Build history of the part. All positions in model axes, mm. A direction names the side the tool comes from. Coordinates: 2 decimals unless noted, no trailing zeros. Order: outer loops, then holes, each group sorted by start corner. A loop starts at its lowest first (then second) coordinate and runs counter-clockwise, first axis right, second up. Notation, with made-up numbers: (85.25, 30.25) -> (102.25, 30.25) arc R29 cw to (102.25, 63.25) -> close; hole circle Ø3 at (25.25, -8). An arc over 180 degrees is marked (long way). Write each question's results on one line, items separated by ' | '.
from build123d import *

# Parameters (mm, degrees)
F1_DEPTH      = 25.4
F1_DEPTH_BACK = 25.4
F2_W          = 21.4085327461
F2_H          = 21.4085327461
F3_DEPTH      = 25.4


with BuildPart() as f1:
    # F0 (on Front) → F1 (new body, two sides)
    with BuildSketch(Plane.XZ) as f1_sk:
        Polygon((0, 48.854034394), (0, 0), (77.7433076873, 0), (77.7433076873, 48.854034394), (56.3347749412, 48.854034394), (56.3347749412, 13.927792199), (21.4085327461, 13.927792199), (21.4085327461, 48.854034394), align=None)
    extrude(amount=F1_DEPTH)
    extrude(f1_sk.sketch, amount=-F1_DEPTH_BACK)

    # F2 (on face) → F3 (cut)
    with BuildSketch(Plane.XY.offset(48.854034394)):
        with Locations((67.0390413143, -2.2439309396)):
            Rectangle(F2_W, F2_H)
    extrude(amount=-F3_DEPTH, mode=Mode.SUBTRACT)


solid = f1.part
Item 1: Slice it at C-C, the plane x = 64.5. List the corners of the cut face in (y, z).
Answer:
outline: (-25.4, 0) -> (25.4, 0) -> (25.4, 48.85) -> (8.46, 48.85) -> (8.46, 23.45) -> (-12.95, 23.45) -> (-12.95, 48.85) -> (-25.4, 48.85) -> close
Item 2: Tool access for faces 4 (the flat face through (67, -12.948, 36)), 5 (the flat face through (21.409, 0, 31)), 6 (the flat face through (0, 0, 25)): list every direction of +Z, -Z, +X, -X, +Y, -Y with a clear straight run to the whole face (end or side of a thin tool).
Answer:
face 4: +Z, +X | face 5: +Z, +Y, -Y | face 6: +Z, -Z, -X, +Y, -Y
Item 3: Slice it at B-B, the plane z = 45. List the corners of the cut face in (x, y), and give its area (3 significant figures).
Answer:
outline: (0, -25.4) -> (21.41, -25.4) -> (21.41, 25.4) -> (0, 25.4) -> close; (56.33, -25.4) -> (77.74, -25.4) -> (77.74, -12.95) -> (56.33, -12.95) -> close; (56.33, 8.46) -> (77.74, 8.46) -> (77.74, 25.4) -> (56.33, 25.4) -> close | area: 1,720 mm^2
Item 4: Slice it at A-A, the plane z = 16. List the corners of the cut face in (x, y), and give its area (3 significant figures).
Answer:
outline: (0, -25.4) -> (21.41, -25.4) -> (21.41, 25.4) -> (0, 25.4) -> close; (56.33, -25.4) -> (77.74, -25.4) -> (77.74, 25.4) -> (56.33, 25.4) -> close | area: 2,180 mm^2
Item 5: Pull direction X, two halves, no side cores. Call faces 1 (the flat face through (56.335, 0, 20)), 2 (the flat face through (77.743, 0, 19)), 3 (the flat face through (38, -25.4, 8)): released by +X, released by -X, zero draft, split by the parting line, or undercut.
Answer:
face 1: undercut | face 2: released by +X | face 3: zero draft
Item 6: Drill centre lines: line 1 (X direction, y = -4.5, z = 19.5); line 2 (Y direction, x = 69, z = 31); line 3 (Z direction, x = 48.5, y = 14). Where is each one in solid material? Low to high. Write a range as from..to.
Answer:
line 1: x = 0..21.41, 56.33..77.74 | line 2: y = -25.4..-12.95, 8.46..25.4 | line 3: z = 0..13.93
Item 7: Slice it at D-D, the plane y = -6. List the corners of the cut face in (x, z).
Answer:
outline: (0, 0) -> (77.74, 0) -> (77.74, 23.45) -> (56.33, 23.45) -> (56.33, 13.93) -> (21.41, 13.93) -> (21.41, 48.85) -> (0, 48.85) -> close
Item 8: Pin check, flat tip, straight feed: pin 1 (1.5 mm diameter, centred on x = 41, y = -8, fed in from +Z). Stop position of the tip, or through.
Answer:
pin 1: stops at z = 13.93
